Verification items for the finished model (mm, model axes). Face numbers are marked on the shaded views. Give positions to 0.01 mm unless a question says otherwise; leave off trailing zeros. Write each loop counter-clockwise with the first axis right and the second up, starting at its lowest first coordinate (ties: lowest second). Pieces come first, ordered by that corner, then holes. Notation, with made-up numbers: (55, 48) -> (93, 48) arc R30 ccw to (93, 71) -> close; hole circle Ø4 at (66.25, -37.5). An arc over 180 degrees is marked (long way). Use CSV: the item, a comma, the result in double quotes. Start each with the question number.
Autodesk Inventor part; units mm, degrees
ref_plane "YZ Plane" through (0, 0, 0) normal (1, 0, 0) x (0, 1, 0)
ref_plane "XZ Plane" through (0, 0, 0) normal (0, 1, 0) x (-1, 0, 0)
ref_plane "XY Plane" through (0, 0, 0) normal (0, 0, 1) x (1, 0, 0)
sketch "Sketch1" plane through (0, 0, 0) normal (1, 0, 0) x (0, 1, 0)
  circle A0 centre (0, 0) radius 10.9
  dimension "d0" = 21.8
extrude "Extrusion1" add sketch "Sketch1" along normal blind 2.6
sketch "Sketch2" plane through (0, 0, 0) normal (-1, 0, 0) x (0, 0, 1)
  circle A0 centre (0, 0) radius 2.5
  circle A1 centre (0, 0) radius 3.5
  dimension "d3" = 5
  dimension "d4" = 7
extrude "Extrusion2" add sketch "Sketch2" along normal blind 2.2
sketch "Sketch3" plane through (2.6, 0, 0) normal (1, 0, 0) x (0, 0, -1)
  circle A0 centre (0, 0) radius 1
  dimension "d7" = 2
hole "Hole1" at (2.6, 0, 0) direction (-1, 0, 0) diameter 2 depth 2
thread "Thread1"
sketch "Sketch4" plane through (2.6, 0, 0) normal (1, 0, 0) x (0, 0, -1)
  circle A0 centre (0, 0) radius 1
  circle A1 centre (0, 0) radius 7
  circle A2 centre (-7, 0) radius 1
  circle A3 centre (0, -7) radius 1
  circle A4 centre (7, 0) radius 1
  circle A5 centre (0, 7) radius 1
  dimension "d17" = 14
  dimension "d18" = 2
  dimension "d21" = 360
hole "Hole2" at (2.6, -7, 0) at (2.6, 0, 7) at (2.6, 7, 0) at (2.6, 0, -7) at (2.6, 0, 0) direction (-1, 0, 0) diameter 2 depth 3
thread "Thread2"
thread "Thread3"
thread "Thread4"
thread "Thread5"
properties part number "Part L"
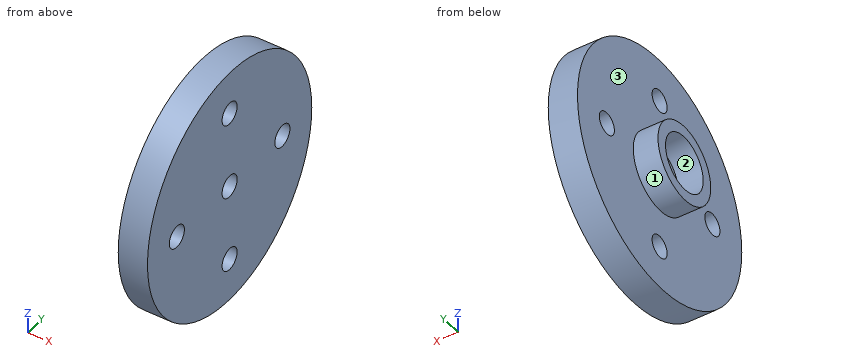
(1) Section check D-D on z = -6.25. Record the cut outline in (x, y).
(2) Go/stop test with flat-tipped pins: pin 1 (3 mm diameter, centred on y = 0, z = -7, fed in from -X); pin 2 (1.5 mm diameter, centred on x = 0.5, z = -4.5, fed in from -Y); pin 3 (1.6 mm diameter, centred on y = -7, z = 0, fed in from +X); pin 4 (1.5 mm diameter, centred on x = 0, z = 7.5, fed in from -Y). Record where each tip stops, or that it passes through.
(3) Section check B-B on y = 0. Record the cut outline in (x, z), then the cut area to 3 significant figures.
(4) Draft check along Y on the marked faces 1, 2 and 3. Enter one of: released by +Y, released by -Y, zero draft, split by the parting line, or undercut.
(5) Section check A-A on x = 0.5. Record the cut outline in (y, z), then the cut area to 3 significant figures.
(6) Thickness scan on line 1 (Y direction, x = -0.9, z = 0); line 2 (Z direction, x = 1.5, y = 0); line 3 (X direction, y = 2.25, z = 7.75). Record the ranges inside material, lowest first. Write a range as from..to.
Data:
1,outline,"(0, -8.93) -> (2.6, -8.93) -> (2.6, -0.66) -> (0, -0.66) -> close; (0, 0.66) -> (2.6, 0.66) -> (2.6, 8.93) -> (0, 8.93) -> close"
2,pin 1,"stops at x = 0"
2,pin 2,"stops at y = -10.23"
2,pin 3,"passes through"
2,pin 4,"stops at y = -8.56"
3,outline,"(-2.2, -3.5) -> (0, -3.5) -> (0, -6) -> (2.6, -6) -> (2.6, -1) -> (0, -1) -> (0, -2.5) -> (-2.2, -2.5) -> close; (-2.2, 2.5) -> (0, 2.5) -> (0, 1) -> (2.6, 1) -> (2.6, 6) -> (0, 6) -> (0, 3.5) -> (-2.2, 3.5) -> close; (0, -10.9) -> (2.6, -10.9) -> (2.6, -8) -> (0, -8) -> close; (0, 8) -> (2.6, 8) -> (2.6, 10.9) -> (0, 10.9) -> close"
3,area,"45.5 mm2"
4,face 1,"split by the parting line"
4,face 2,"undercut"
4,face 3,"zero draft"
5,outline,"circle Ø21.8 at (0, 0); hole circle Ø2 at (-7, 0); hole circle Ø2 at (0, -7); hole circle Ø2 at (0, 0); hole circle Ø2 at (0, 7); hole circle Ø2 at (7, 0)"
5,area,"358 mm2"
6,line 1,"y = -3.5..-2.5, 2.5..3.5"
6,line 2,"z = -10.9..-8, -6..-1, 1..6, 8..10.9"
6,line 3,"x = 0..2.6"
